Geometry check sheet. Reference: the model listing, model coordinates, mm. Give positions to 0.01 mm unless a question says otherwise; leave off trailing zeros. Order: outer loops, then holes, each group sorted by start corner. A loop starts at its lowest first (then second) coordinate and runs counter-clockwise, first axis right, second up. Notation, with made-up numbers: M -22.5,67 L 0.5,67 A9 ccw 0.5,82 Z; hole C -21.5,15.25 d7. An arc over 180 degrees is marked long. Use CSV: the item, a comma, the result in double quotes. Start each with the question number.
from build123d import *

# Parameters (mm, degrees)
BOSS_EXTRUDE1_DEPTH = 10
SKETCH3_R           = 3.75
CUT_EXTRUDE1_DEPTH  = 5
SKETCH4_R           = 3.75
BOSS_EXTRUDE2_DEPTH = 10


with BuildPart() as part:
    # Sketch1 → Boss-Extrude1 (new body)
    with BuildSketch(Plane(origin=(0, 0, 0), x_dir=(1, 0, 0), z_dir=(0, 1, 0))):
        with BuildLine():
            Line((101.452048182, 5.461568526), (4.840160607, 24.526981985))
            ThreePointArc((4.840160607, 24.526981985), (-24.995505199, 0.474046272), (3.906693314, -24.69286835))
            Line((3.906693314, -24.69286835), (101.172007994, -9.304386575))
            ThreePointArc((101.172007994, -9.304386575), (107.49865156, -2.038739951), (101.452048182, 5.461568526))
        make_face()
    extrude(amount=BOSS_EXTRUDE1_DEPTH)

    # Sketch3 → Cut-Extrude1 (cut)
    with BuildSketch(Plane.XZ):
        with Locations((100, 1.89652607)):
            Circle(SKETCH3_R)
        with BuildLine():
            Line((17.529407273, -2.952918523), (1.075988404, -5.902732327))
            ThreePointArc((1.075988404, -5.902732327), (-9e-09, -6), (-1.075988422, -5.902732329))
            Line((-1.075988422, -5.902732329), (-17.529407298, -2.952918565))
            ThreePointArc((-17.529407298, -2.952918565), (-20.000000128, 0), (-17.529407298, 2.952918565))
            Line((-17.529407298, 2.952918565), (-1.075988422, 5.902732329))
            ThreePointArc((-1.075988422, 5.902732329), (-9e-09, 6), (1.075988404, 5.902732327))
            Line((1.075988404, 5.902732327), (17.529407273, 2.952918523))
            ThreePointArc((17.529407273, 2.952918523), (19.999999872, 0), (17.529407273, -2.952918523))
        make_face()
    extrude(amount=-CUT_EXTRUDE1_DEPTH, mode=Mode.SUBTRACT)

    # Sketch4 → Boss-Extrude2 (add)
    with BuildSketch(Plane.XZ.offset(-5)):
        with Locations((100, 1.89652607)):
            Circle(SKETCH4_R)
    extrude(amount=BOSS_EXTRUDE2_DEPTH)


solid = part.part
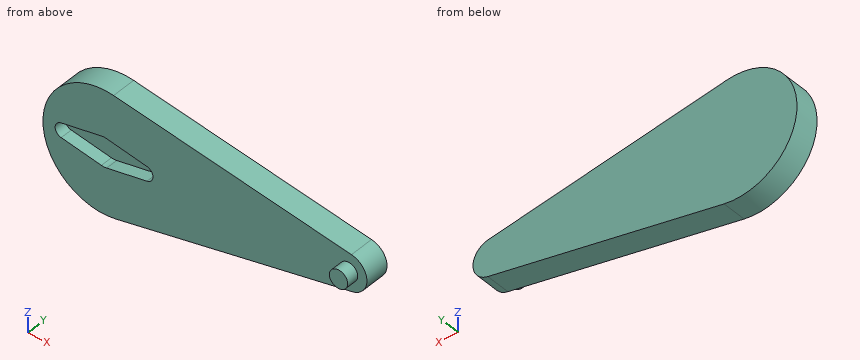
(1) Go/stop test with flat-tipped pins: P1, Ø5, axis at x = 68.5, z = -11.5, coming from the -Y side; P2, Ø8, axis at x = 23.5, y = 7, coming from the -Z side; P3, Ø3, axis at y = 5.5, z = -3, coming from the +X side. Record where each tip stops, or that it passes through.
(2) Sectioned sample at A-A on y = 2.25. Record the cut outline in (x, z), then the cut area to 3 significant figures.
(3) Thickness scan on line 1 (Y direction, x = 72.5, z = 1.5); line 2 (Y direction, x = 1, z = 4.5); line 3 (Z direction, x = -0.5, y = 9) (3 decimals). Record the ranges inside material, lowest first.
(4) Sectioned sample at C-C on x = 100. Record the cut outline in (y, z), then the cut area to 3 significant figures.
(5) Sectioned sample at D-D on y = 8. Record the cut outline in (x, z), then the cut area to 3 significant figures.
(6) Sectioned sample at B-B on z = 0. Record the cut outline in (x, y).
Responses:
1,P1,"y = 0"
1,P2,"z = -21.63"
1,P3,"x = 106.69"
2,outline,"M 3.91,24.69 A25 ccw long 4.84,-24.53 L 101.45,-5.46 A7.5 ccw 101.17,9.3 Z; hole M -17.53,-2.95 L -1.08,-5.9 A6 ccw 1.08,-5.9 L 17.53,-2.95 A3 ccw 17.53,2.95 L 1.08,5.9 A6 ccw -1.08,5.9 L -17.53,2.95 A3 ccw Z"
2,area,"4,030 mm2"
3,line 1,"0 to 10"
3,line 2,"5 to 10"
3,line 3,"-24.995 to 24.995"
4,outline,"M -5,-1.85 L 0,-1.85 L 0,-5.75 L 10,-5.75 L 10,9.49 L 0,9.49 L 0,5.65 L -5,5.65 Z"
4,area,"190 mm2"
5,outline,"M 3.91,24.69 A25 ccw long 4.84,-24.53 L 101.45,-5.46 A7.5 ccw 101.17,9.3 Z"
5,area,"4,370 mm2"
6,outline,"M -25,0 L -20,0 L -20,5 L 20,5 L 20,0 L 96.76,0 L 96.76,-5 L 103.24,-5 L 103.24,0 L 107.26,0 L 107.26,10 L -25,10 Z"
